```python
from build123d import *

# Parameters (mm, degrees)
SKETCH1_R           = 1.609204822
BOSS_EXTRUDE1_DEPTH = 3
SKETCH2_W           = 39.09
SKETCH2_H           = 79.17
CUT_EXTRUDE1_DEPTH  = 67.15748257


with BuildPart() as part:
    # Sketch1 → Boss-Extrude1 (new body)
    with BuildSketch(Plane(origin=(0, 0, 0), x_dir=(1, 0, 0), z_dir=(0, 1, 0))):
        Polygon((-30.75, 58.5), (-30.75, 19.5), (-27.75, 19.5), (-27.75, -19.5), (-30.75, -19.5), (-30.75, -58.5), (-14, -58.5), (-14, -55.5), (14, -55.5), (14, -58.5), (30.75, -58.5), (30.75, -19.5), (27.75, -19.5), (27.75, 19.5), (30.75, 19.5), (30.75, 58.5), (14, 58.5), (14, 55.5), (-14, 55.5), (-14, 58.5), align=None)
        with Locations(Location((-22, -42.94, 0), (0, 0, 270))):
            Circle(SKETCH1_R, mode=Mode.SUBTRACT)
        with Locations(Location((22, -42.94, 0), (0, 0, 270))):
            Circle(SKETCH1_R, mode=Mode.SUBTRACT)
        with Locations(Location((22, 42.94, 0), (0, 0, 270))):
            Circle(SKETCH1_R, mode=Mode.SUBTRACT)
        with Locations(Location((-22, 42.94, 0), (0, 0, 270))):
            Circle(SKETCH1_R, mode=Mode.SUBTRACT)
    extrude(amount=BOSS_EXTRUDE1_DEPTH)

    # Sketch2 → Cut-Extrude1 (cut, through all)
    with BuildSketch(Plane(origin=(0, 3, 0), x_dir=(1, 0, 0), z_dir=(0, 1, 0))):
        Rectangle(SKETCH2_W, SKETCH2_H)
    extrude(amount=-CUT_EXTRUDE1_DEPTH, mode=Mode.SUBTRACT)


solid = part.part
```
Design review of the part built by this model. Coordinates are the model's own, in mm. A direction names the side the tool comes from. Round coordinates to 2 decimals unless told otherwise and drop trailing zeros. Order: outer loops, then holes, each group sorted by start corner. A loop starts at its lowest first (then second) coordinate and runs counter-clockwise, first axis right, second up. Notation, with made-up numbers: M -5.75,-16.75 L 38.25,-16.75 A15 cw 38.25,-3.75 Z; hole C 87,32 d9. An arc over 180 degrees is marked long. Put each result on its own line as item: value.
Q1. Consider section D-D (z = -42.94). State the section outline as (x, y) points, and give its area (3 significant figures).
Reported:
outline: M -30.75,0 L -23.61,0 L -23.61,3 L -30.75,3 Z; M -20.39,0 L 20.39,0 L 20.39,3 L -20.39,3 Z; M 23.61,0 L 30.75,0 L 30.75,3 L 23.61,3 Z
area: 165 mm²
Q2. Insertion check: pin 1 Ø1.5 at (x, y) = (-4.5, 1.5) entering from +Z; pin 2 Ø0.9 at (x, y) = (-2, 1) entering from -Z. Each pin has a flat end and moves straight along its axis. Give the tip position at first contact, or say it passes through.
Reported:
pin 1: z = 55.5
pin 2: z = -55.5
Q3. To check wall thickness, follow line 1 (X direction, y = 2.05, z = 42.94); line 2 (Z direction, x = -2, y = 2.05) (3 decimals); line 3 (X direction, y = 1.7, z = 25.5) (3 decimals). State the ranges of each line that lie inside material, in increasing order.
Reported:
line 1: -30.75 to -23.61, -20.39 to 20.39, 23.61 to 30.75
line 2: -55.5 to -39.585, 39.585 to 55.5
line 3: -30.75 to -19.545, 19.545 to 30.75
Q4. Consider section B-B (z = -12). State the section outline as (x, y) points (3 decimals).
Reported:
outline: M -27.75,0 L -19.545,0 L -19.545,3 L -27.75,3 Z; M 19.545,0 L 27.75,0 L 27.75,3 L 19.545,3 Z
Q5. Draft analysis for pull direction Z (two halves, no side actions). For faces 6 (the face through (22, 1, 58.5)), 7 (the face through (-27.75, 1, 0)), 8 (the face through (30.75, 1, 39)), state which applies: released by +Z, released by -Z, zero draft, split by the parting line, or undercut.
Reported:
face 6: released by +Z
face 7: undercut
face 8: zero draft
Q6. Machinability: for faces 1 (the face through (29, 1, 19.5)), 2 (the face through (0, 1, 55.5)), 3 (the face through (-29, 1, -19.5)), 4 (the face through (0, 1, -55.5)), 5 (the face through (19.545, 2, 1)), which of the approach directions +Z, -Z, +X, -X, +Y, -Y give a long, thin tool a straight path to every point of the face, cutting with its end or side? Answer none if there is none.
Reported:
face 1: +X, +Y, -Y
face 2: +Z, +Y, -Y
face 3: -X, +Y, -Y
face 4: -Z, +Y, -Y
face 5: +Y, -Y
Q7. Consider section C-C (y = 0.5). State the section outline as (x, z) points (3 decimals).
Reported:
outline: M -30.75,-58.5 L -14,-58.5 L -14,-55.5 L 14,-55.5 L 14,-58.5 L 30.75,-58.5 L 30.75,-19.5 L 27.75,-19.5 L 27.75,19.5 L 30.75,19.5 L 30.75,58.5 L 14,58.5 L 14,55.5 L -14,55.5 L -14,58.5 L -30.75,58.5 L -30.75,19.5 L -27.75,19.5 L -27.75,-19.5 L -30.75,-19.5 Z; hole C -22,-42.94 d3.218; hole C -22,42.94 d3.218; hole M -19.545,-39.585 L 19.545,-39.585 L 19.545,39.585 L -19.545,39.585 Z; hole C 22,-42.94 d3.218; hole C 22,42.94 d3.218
Q8. Consider section A-A (x = 7.5). State the section outline as (y, z) points (3 decimals), and give its area (3 significant figures).
Reported:
outline: M 0,-55.5 L 3,-55.5 L 3,-39.585 L 0,-39.585 Z; M 0,39.585 L 3,39.585 L 3,55.5 L 0,55.5 Z
area: 95.5 mm²
